Verification items for this drawing (mm, ordinates from the low corner). A direction names the side the tool comes from. Coordinates: 2 decimals unless noted, no trailing zeros. Order: outer loops, then holes, each group sorted by start corner. A loop starts at its lowest first (then second) coordinate and runs counter-clockwise, first axis right, second up. Notation, with made-up numbers: M 20,-17.75 L 26,-17.75 A23 ccw 26,7.25 Z; hole C 51,43.5 d5. An arc over 180 degrees is marked long. Answer as a JSON object with one key per item and string values. Group by question number.
(1) Cross-section at D-D (z = 0.5). Enter the section's corners in (x, y).
(2) Cross-section at B-B (x = 17.1). Enter the section's corners in (y, z).
(3) Cross-section at A-A (y = 3.5). Enter the section's corners in (x, z).
(4) Access from +Z, -Z, +X, -X, +Y, -Y to the whole of each face (thin tool, end or side, straight path). Record for the marked faces 1, 2, 3, 4 and 5.
(5) Gauge pin test, flat ends, axial feed: pin 1 Ø0.8 at (y, z) = (6, 1.5) entering from -X; pin 2 Ø1 at (x, z) = (1.3, 1.3) entering from -Y; pin 3 Ø0.8 at (x, z) = (1, 1.5) entering from +Y; pin 4 Ø1.3 at (x, z) = (17, 1) entering from +Y. Record the tip position at first contact, or that the pin passes through.
(6) Cross-section at C-C (z = 1.3). Enter the section's corners in (x, y).
(7) Material ranges on line 1 (X direction, y = 1.25, z = 1.3); line 2 (X direction, y = 8, z = 2.1); line 3 (Z direction, x = 17.1, y = 0.75), recorded low to high.
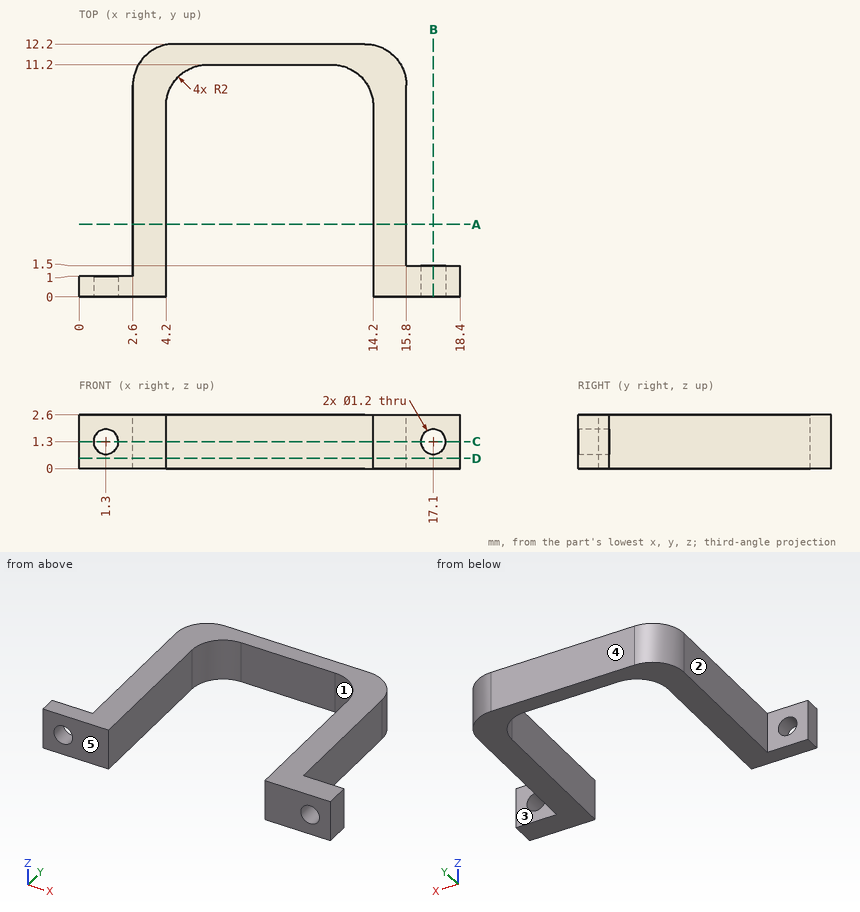
Taken from the geometry:
{
 "1": {"outline": "M 0,0 L 4.2,0 L 4.2,9.2 A2 cw 6.2,11.2 L 12.2,11.2 A2 cw 14.2,9.2 L 14.2,0 L 18.4,0 L 18.4,1.5 L 15.8,1.5 L 15.8,10.2 A2 ccw 13.8,12.2 L 4.6,12.2 A2 ccw 2.6,10.2 L 2.6,1 L 0,1 Z"},
 "2": {"outline": "M 0,0 L 1.5,0 L 1.5,0.7 L 0,0.7 Z; M 0,1.9 L 1.5,1.9 L 1.5,2.6 L 0,2.6 Z"},
 "3": {"outline": "M 2.6,0 L 4.2,0 L 4.2,2.6 L 2.6,2.6 Z; M 14.2,0 L 15.8,0 L 15.8,2.6 L 14.2,2.6 Z"},
 "4": {"face 1": "+Z, -Z, -Y", "face 2": "+Z, -Z, -X, +Y", "face 3": "+Z, -Z, +X, +Y", "face 4": "+Z, -Z, +X, -X, +Y", "face 5": "+Z, -Z, +X, -X, -Y"},
 "5": {"pin 1": "stops at x = 2.6", "pin 2": "passes through", "pin 3": "stops at y = 1", "pin 4": "stops at y = 1.5"},
 "6": {"outline": "M 0,0 L 0.7,0 L 0.7,1 L 0,1 Z; M 1.9,0 L 4.2,0 L 4.2,9.2 A2 cw 6.2,11.2 L 12.2,11.2 A2 cw 14.2,9.2 L 14.2,0 L 16.5,0 L 16.5,1.5 L 15.8,1.5 L 15.8,10.2 A2 ccw 13.8,12.2 L 4.6,12.2 A2 ccw 2.6,10.2 L 2.6,1 L 1.9,1 Z; M 17.7,0 L 18.4,0 L 18.4,1.5 L 17.7,1.5 Z"},
 "7": {"line 1": "x = 2.6 to 4.2, 14.2 to 16.5, 17.7 to 18.4", "line 2": "x = 2.6 to 4.2, 14.2 to 15.8", "line 3": "z = 0 to 0.7, 1.9 to 2.6"}
}
